Model file for the job. Use its own axes, mm. A direction names the side the tool comes from. Round coordinates to 2 decimals unless told otherwise and drop trailing zeros. Order: outer loops, then holes, each group sorted by start corner. A loop starts at its lowest first (then second) coordinate and runs counter-clockwise, first axis right, second up. Notation, with made-up numbers: (51.5, 4) -> (97.5, 4) arc R11 ccw to (97.5, 14) -> close; hole circle Ø2 at (-19.5, -13.75). An arc over 180 degrees is marked (long way). Answer as CSV lines item,"result".
```python
from build123d import *

# Parameters (mm, degrees)
SKETCH1_R           = 26
BOSS_EXTRUDE1_DEPTH = 5
SKETCH11_R          = 3
CUT_EXTRUDE7_DEPTH  = 38.107950631
BOSS_EXTRUDE4_START = -5
SKETCH4_R           = 16
BOSS_EXTRUDE4_DEPTH = 30
SKETCH10_W          = 18
SKETCH10_H          = 18
CUT_EXTRUDE8_DEPTH  = 24.25


with BuildPart() as part:
    # Sketch1 → Boss-Extrude1 (new body)
    with BuildSketch(Plane(origin=(0, 0, 0), x_dir=(1, 0, 0), z_dir=(0, 1, 0))):
        with Locations(Location((0, 0, 0), (0, 0, 270))):
            Circle(SKETCH1_R)
    extrude(amount=BOSS_EXTRUDE1_DEPTH)

    # Sketch11 → Cut-Extrude7 (cut, through all)
    with BuildSketch(Plane(origin=(0, 5, 0), x_dir=(1, 0, 0), z_dir=(0, 1, 0))):
        with Locations(Location((-16.454482672, -9.5, 0), (0, 0, 270))):
            Circle(SKETCH11_R)
        with Locations(Location((-16.454482672, 9.5, 0), (0, 0, 270))):
            Circle(SKETCH11_R)
        with Locations(Location((0, 19, 0), (0, 0, 270))):
            Circle(SKETCH11_R)
        with Locations(Location((16.454482672, 9.5, 0), (0, 0, 270))):
            Circle(SKETCH11_R)
        with Locations(Location((16.454482672, -9.5, 0), (0, 0, 270))):
            Circle(SKETCH11_R)
        with Locations(Location((0, -19, 0), (0, 0, 270))):
            Circle(SKETCH11_R)
    extrude(amount=-CUT_EXTRUDE7_DEPTH, mode=Mode.SUBTRACT)

    # Sketch4 → Boss-Extrude4 (add)
    with BuildSketch(Plane(origin=(0, 5, 0), x_dir=(1, 0, 0), z_dir=(0, 1, 0)).offset(BOSS_EXTRUDE4_START)):
        with Locations(Location((0, 0, 0), (0, 0, 270))):
            Circle(SKETCH4_R)
    extrude(amount=-BOSS_EXTRUDE4_DEPTH)

    # Sketch10 → Cut-Extrude8 (cut)
    with BuildSketch(Plane.XZ.offset(30)):
        Rectangle(SKETCH10_W, SKETCH10_H)
    extrude(amount=-CUT_EXTRUDE8_DEPTH, mode=Mode.SUBTRACT)


solid = part.part
```
Q1. Saw through at C-C (z = -11). Write the cut outline in (x, y), plus the area to 3 significant figures.
Checks:
outline,"(-23.56, 0) -> (-19.05, 0) -> (-19.05, 5) -> (-23.56, 5) -> close; (-13.86, 0) -> (-11.62, 0) -> (-11.62, -30) -> (11.62, -30) -> (11.62, 0) -> (13.86, 0) -> (13.86, 5) -> (-13.86, 5) -> close; (19.05, 0) -> (23.56, 0) -> (23.56, 5) -> (19.05, 5) -> close"
area,"881 mm²"
Q2. Saw through at B-B (y = -11). Write the cut outline in (x, z), plus the area to 3 significant figures.
Checks:
outline,"circle Ø32 at (0, 0); hole (-9, -9) -> (9, -9) -> (9, 9) -> (-9, 9) -> close"
area,"480 mm²"
Q3. Mould opens along Z. For faces 3 (the cylindrical face through (-14.427, 2.535, -11.711)), 4 (the flat face through (0, 5, 0)), 5 (the cylindrical face through (-15.62, -14.79, -3.47)) say: +Z half, -Z half, draft (parallel to the pull), parting line (faces both ways), or undercut.
Checks:
face 3,"undercut"
face 4,"draft"
face 5,"parting line"
Q4. Saw through at A-A (z = -18.5). Write the cut outline in (x, y).
Checks:
outline,"(-18.27, 0) -> (-2.96, 0) -> (-2.96, 5) -> (-18.27, 5) -> close; (2.96, 0) -> (18.27, 0) -> (18.27, 5) -> (2.96, 5) -> close"
Q5. Wall check: L1, parallel to X at y = -15, z = 0.5; L2, parallel to Z at x = 16, y = 0.5; L3, parallel to Z at x = -15, y = 3. Give the ranges that are in metal, low to high. Write a range as [from, to].
Checks:
L1,"[-15.99, -9], [9, 15.99]"
L2,"[-20.49, -12.47], [-6.53, 6.53], [12.47, 20.49]"
L3,"[-21.24, -12.12], [-6.88, 6.88], [12.12, 21.24]"
Q6. Tool access for faces 1 (the cylindrical face through (-15.821, 2.465, -20.633)), 2 (the flat face through (9, -18, 0)): list every direction of +Z, -Z, +X, -X, +Y, -Y with a clear straight run to the whole face (end or side of a thin tool).
Checks:
face 1,"+Y, -Y"
face 2,"-Y"
Q7. Flat gauge pins, fed straight in: pin 1 (9.5 mm diameter, centred on x = -16.45, z = 9.5, fed in from -Y); pin 2 (20 mm diameter, centred on y = -17.5, z = 4, fed in from +X); pin 3 (14.5 mm diameter, centred on x = 0.5, y = -19.5, fed in from -Z); pin 4 (9 mm diameter, centred on x = -3.5, y = -18.5, fed in from +Z). Where does each tip first touch, or does it go through?
Checks:
pin 1,"y = -30"
pin 2,"x = 16"
pin 3,"z = -16"
pin 4,"z = 16"
Q8. Saw through at D-D (y = 3). Write the cut outline in (x, z).
Checks:
outline,"circle Ø52 at (0, 0); hole circle Ø6 at (-16.45, -9.5); hole circle Ø6 at (-16.45, 9.5); hole circle Ø6 at (0, -19); hole circle Ø6 at (0, 19); hole circle Ø6 at (16.45, -9.5); hole circle Ø6 at (16.45, 9.5)"
